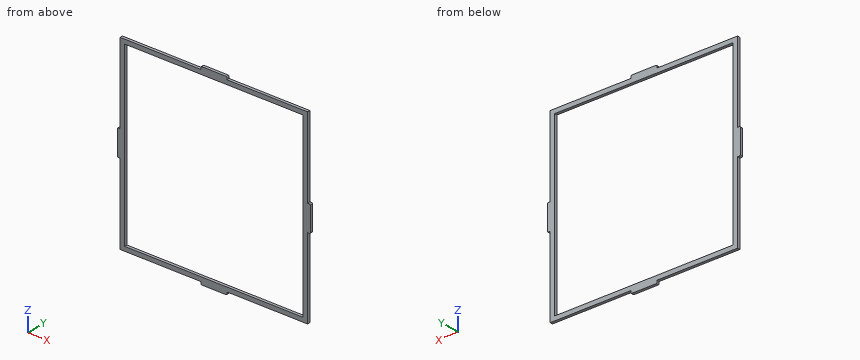
```python
from build123d import *

# Parameters (mm, degrees)
SKETCH1_W           = 215.91
SKETCH1_H           = 215.91
BOSS_EXTRUDE1_DEPTH = 3.175
SKETCH2_W           = 205.91
SKETCH2_H           = 205.91
CUT_EXTRUDE1_DEPTH  = 4.175
SKETCH4_W           = 3.175
SKETCH4_H           = 30
SKETCH4_W_2         = 30
SKETCH4_H_2         = 3.175
BOSS_EXTRUDE2_DEPTH = 3.175
FILLET1_R           = 1


with BuildPart() as part:
    # Sketch1 → Boss-Extrude1 (new body)
    with BuildSketch(Plane(origin=(0, 0, 0), x_dir=(1, 0, 0), z_dir=(0, 1, 0))):
        Rectangle(SKETCH1_W, SKETCH1_H)
    extrude(amount=BOSS_EXTRUDE1_DEPTH)

    # Sketch2 → Cut-Extrude1 (cut, through all)
    with BuildSketch(Plane(origin=(0, 3.175, 0), x_dir=(1, 0, 0), z_dir=(0, 1, 0))):
        Rectangle(SKETCH2_W, SKETCH2_H)
    extrude(amount=-CUT_EXTRUDE1_DEPTH, mode=Mode.SUBTRACT)

    # Sketch4 → Boss-Extrude2 (add)
    with BuildSketch(Plane(origin=(0, 3.175, 0), x_dir=(1, 0, 0), z_dir=(0, 1, 0))):
        with Locations((-109.5425, 0)):
            Rectangle(SKETCH4_W, SKETCH4_H)
        with Locations((0, 109.5425)):
            Rectangle(SKETCH4_W_2, SKETCH4_H_2)
        with Locations((0, -109.5425)):
            Rectangle(SKETCH4_W_2, SKETCH4_H_2)
        with Locations((109.5425, 0)):
            Rectangle(SKETCH4_W, SKETCH4_H)
    extrude(amount=-BOSS_EXTRUDE2_DEPTH)

    # Fillet1
    fillet1_edges = [part.edges().sort_by_distance(p)[0] for p in [
        (-111.13, 1.5875, 15),
        (-111.13, 1.5875, -15),
        (-15, 1.5875, 111.13),
        (15, 1.5875, 111.13),
        (-15, 1.5875, -111.13),
        (15, 1.5875, -111.13),
        (111.13, 1.5875, 15),
        (111.13, 1.5875, -15),
    ]]
    fillet(fillet1_edges, radius=FILLET1_R)


solid = part.part
```
Model file for the job. Use its own axes, mm. Coordinates: 2 decimals unless noted, no trailing zeros. Order: outer loops, then holes, each group sorted by start corner. A loop starts at its lowest first (then second) coordinate and runs counter-clockwise, first axis right, second up. Notation, with made-up numbers: (71.25, 76.25) -> (88.25, 76.25) arc R18 cw to (88.25, 95.25) -> close; hole circle Ø3 at (-23, 69.5). An arc over 180 degrees is marked (long way). Return JSON: item names as keys, results as strings.
Item 1: Wall check: line 1 along Z through (x, y) = (7, 2.3) (3 decimals); line 2 along Z through (x, y) = (81, 1.85) (3 decimals). Give the ranges that are in metal, low to high. Write a range as from..to.
Model answer:
{"line 1": "z = -111.13..-102.955, 102.955..111.13", "line 2": "z = -107.955..-102.955, 102.955..107.955"}
Item 2: Slice it at A-A (x = 28). Write the cut outline in (y, z) (3 decimals), then the cut area to 4 significant figures.
Model answer:
{"outline": "(0, -107.955) -> (3.175, -107.955) -> (3.175, -102.955) -> (0, -102.955) -> close; (0, 102.955) -> (3.175, 102.955) -> (3.175, 107.955) -> (0, 107.955) -> close", "area": "31.75 mm²"}
Item 3: Pin check, flat tips, straight feed: P1, Ø1.7, axis at x = 108.5, y = 1.5, coming from the -Z side (3 decimals); P2, Ø1.5, axis at x = -27.5, y = 2, coming from the +Z side (3 decimals); P3, Ø1, axis at y = 1, z = -47, coming from the -X side (3 decimals). Stop position of each tip, or through.
Model answer:
{"P1": "stops at z = -107.955", "P2": "stops at z = 107.955", "P3": "stops at x = -107.955"}
Item 4: Slice it at B-B (z = -2). Write the cut outline in (x, y) (3 decimals), then the cut area to 3 significant figures.
Model answer:
{"outline": "(-111.13, 0) -> (-102.955, 0) -> (-102.955, 3.175) -> (-111.13, 3.175) -> close; (102.955, 0) -> (111.13, 0) -> (111.13, 3.175) -> (102.955, 3.175) -> close", "area": "51.9 mm²"}
